from build123d import *

# Parameters (mm, degrees)
F0_R     = 1
F1_DEPTH = 5.3
F3_R     = 1.95
F4_DEPTH = 1
F6_W     = 0.61
F6_H     = 1.82
F7_DEPTH = 0.5
F8_R     = 0.6


with BuildPart() as f1:
    # F0 (on Front) → F1 (new body)
    with BuildSketch(Plane.XZ):
        Circle(F0_R)
    extrude(amount=F1_DEPTH)

    # F3 (on offset) → F4 (join)
    with BuildSketch(Plane.XZ.offset(5.3)):
        Circle(F3_R)
    extrude(amount=F4_DEPTH)

    # F6 (on offset) → F7 (cut)
    with BuildSketch(Plane.XZ.offset(6.3)):
        Rectangle(F6_W, F6_H)
    extrude(amount=-F7_DEPTH, mode=Mode.SUBTRACT)

    # F8
    f8_edges = [f1.edges().sort_by_distance(p)[0] for p in [
        (-1.95, -6.3, 0),
    ]]
    fillet(f8_edges, radius=F8_R)


solid = f1.part
Work out the finished part from the listing and answer in its coordinate system (mm). A direction names the side the tool comes from. Coordinates: 2 decimals unless noted, no trailing zeros. Write each loop counter-clockwise with the first axis right and the second up, starting at its lowest first coordinate (ties: lowest second). Pieces come first, ordered by that corner, then holes. Notation, with made-up numbers: M 56,75.25 L 114,75.25 A19 ccw 114,87.25 Z; hole C 52,-19 d7. An arc over 180 degrees is marked long. Use one line per item in the form item = value. Start each with the question number.
1. Straight lines are drawn through the part: probe 1 along Y at (x, z) = (-0.2, 1.3); probe 2 along Y at (x, z) = (0.05, 0.75); probe 3 along Z at (x, y) = (-0.4, -5). For each, find the intervals that lie inside material, in ascending order. Write a range as from..to.
2. The part is cut by section C-C (y = -4). Give the vertices of the cut face in (x, z), plus the area to 3 significant figures.
3. A tool of negligible diameter and unlimited length cuts with its end or side. For faces 1 (the face through (1, -5.3, -1)), 2 (the face through (-1.437, -5.497, 1.318)), from which of +Z, -Z, +X, -X, +Y, -Y can it reach the whole face along a straight path? Write none if from no direction.
4. The part is cut by section D-D (y = -6). Give the vertices of the cut face in (x, z) (3 decimals), plus the area to 3 significant figures.
5. The part is cut by section A-A (x = 0). Give the vertices of the cut face in (y, z).
6. The part is cut by section B-B (z = 0). Give the vertices of the cut face in (x, y) (3 decimals).
7. This flat-tipped pin is pushed along its axis until it touches: P1, Ø1.5, axis at x = -1, y = -3, coming from the -Z side. Where does it stop, or does it pass through?
Evaluation:
q1.probe_1 = -6.3..-5.3
q1.probe_2 = -5.8..0
q1.probe_3 = -0.92..0.92
q2.outline = C 0,0 d2
q2.area = 3.14 mm^2
q3.face_1 = +Y
q3.face_2 = +Y, -Y
q4.outline = C 0,0 d3.739; hole M -0.305,-0.91 L 0.305,-0.91 L 0.305,0.91 L -0.305,0.91 Z
q4.area = 9.87 mm^2
q5.outline = M -6.3,-1.35 A0.6 ccw -5.7,-1.95 L -5.3,-1.95 L -5.3,-1 L 0,-1 L 0,1 L -5.3,1 L -5.3,1.95 L -5.7,1.95 A0.6 ccw -6.3,1.35 L -6.3,0.91 L -5.8,0.91 L -5.8,-0.91 L -6.3,-0.91 Z
q6.outline = M -1.95,-5.7 A0.6 ccw -1.35,-6.3 L -0.305,-6.3 L -0.305,-5.8 L 0.305,-5.8 L 0.305,-6.3 L 1.35,-6.3 A0.6 ccw 1.95,-5.7 L 1.95,-5.3 L 1,-5.3 L 1,0 L -1,0 L -1,-5.3 L -1.95,-5.3 Z
q7.P1 = -0.97
